Could you check a few things on this model? Use its own coordinates, in mm. Face numbers are marked on the shaded views. A direction names the side the tool comes from. Give positions to 0.01 mm unless a question says otherwise; leave off trailing zeros. Write each loop counter-clockwise with the first axis right and the second up, starting at its lowest first coordinate (ties: lowest second). Pieces come first, ordered by that corner, then holes. Notation, with made-up numbers: (11.25, 68) - (53.25, 68) arc R19 cw to (53.25, 96) - close; hole circle Ø3 at (80.25, 44.25). An arc over 180 degrees is marked (long way). Write item = value, one per line.
from build123d import *

# Parameters (mm, degrees)
SKETCH1_R           = 1.6
BOSS_EXTRUDE1_DEPTH = 5
BOSS_EXTRUDE2_DEPTH = 79.5
SKETCH3_R           = 11.1
CUT_EXTRUDE1_DEPTH  = 112.08808442
BOSS_EXTRUDE3_START = 3
SKETCH4_R           = 15
SKETCH4_R_2         = 11.1
BOSS_EXTRUDE3_DEPTH = 3
CHAMFER1_SIZE       = 3
BOSS_EXTRUDE4_START = -1
SKETCH5_R           = 11.1
SKETCH5_R_2         = 9.1
BOSS_EXTRUDE4_DEPTH = 1
CHAMFER2_SIZE       = 10
CHAMFER2_SIZE_2     = 0.5
SKETCH6_R           = 1.6
CUT_EXTRUDE2_DEPTH  = 112.08808442
SKETCH7_R           = 11.1
SKETCH7_R_2         = 1.6
CUT_EXTRUDE3_DEPTH  = 112.995814654
BOSS_EXTRUDE5_START = -1
SKETCH8_R           = 11.1
SKETCH8_R_2         = 9.1
BOSS_EXTRUDE5_DEPTH = 1
CHAMFER3_SIZE       = 10
CHAMFER3_SIZE_2     = 0.5
BOSS_EXTRUDE6_START = 5.5
SKETCH9_R           = 1.6
SKETCH9_R_2         = 11.1
BOSS_EXTRUDE6_DEPTH = 5.5
SKETCH10_R          = 12.5
CUT_EXTRUDE4_DEPTH  = 2.5
CHAMFER6_SIZE       = 1
CHAMFER5_SIZE       = 5.5
FILLET4_R           = 5
FILLET5_R           = 5
FILLET6_R           = 5
FILLET7_R           = 5
FILLET1_R           = 10


# Some blends are built 0.0001 mm under size
with BuildPart() as part:
    # Sketch1 → Boss-Extrude1 (new body)
    with BuildSketch(Plane.XY):
        with BuildLine():
            Line((-32.25, -32.25), (-16.996827309, -32.25))
            ThreePointArc((-16.996827309, -32.25), (-13.644608083, -30.959801378), (-12.022400308, -27.755050505))
            ThreePointArc((-12.022400308, -27.755050505), (0.783748237, -0.783748237), (27.755050505, 12.022400308))
            ThreePointArc((27.755050505, 12.022400308), (30.959801378, 13.644608083), (32.25, 16.996827309))
            Line((32.25, 16.996827309), (32.25, 32.25))
            Line((32.25, 32.25), (-32.25, 32.25))
            Line((-32.25, 32.25), (-32.25, -32.25))
        make_face()
        with Locations((-19.75, 19.75)):
            Circle(SKETCH1_R, mode=Mode.SUBTRACT)
        with Locations((-5.65, 19.75)):
            Circle(SKETCH1_R, mode=Mode.SUBTRACT)
        with Locations((25.65, 19.75)):
            Circle(SKETCH1_R, mode=Mode.SUBTRACT)
        with Locations((-19.75, 5.65)):
            Circle(SKETCH1_R, mode=Mode.SUBTRACT)
        with Locations((-19.75, -25.65)):
            Circle(SKETCH1_R, mode=Mode.SUBTRACT)
    extrude(amount=BOSS_EXTRUDE1_DEPTH)

    # Sketch2 → Boss-Extrude2 (add)
    with BuildSketch(Plane.XY.offset(5)):
        Polygon((-32.25, 32.25), (32.25, 32.25), (32.25, 27.25), (-27.25, 27.25), (-27.25, -32.25), (-32.25, -32.25), (-32.25, 27.25), align=None)
    extrude(amount=BOSS_EXTRUDE2_DEPTH)

    # Sketch3 → Cut-Extrude1 (cut, through all)
    with BuildSketch(Plane(origin=(0, 32.25, 0), x_dir=(1, 0, 0), z_dir=(0, 1, 0))):
        with Locations(Location((11.85, -64.1, 0), (0, 0, 270))):
            Circle(SKETCH3_R)
        with BuildLine():
            Line((11.85, -84.5), (11.85, -91.476631288))
            Line((11.85, -91.476631288), (44.100409765, -91.476631288))
            Line((44.100409765, -91.476631288), (44.100409765, -64.1))
            Line((44.100409765, -64.1), (32.25, -64.1))
            ThreePointArc((32.25, -64.1), (26.274978336, -78.524978336), (11.85, -84.5))
        make_face()
    extrude(amount=-CUT_EXTRUDE1_DEPTH, mode=Mode.SUBTRACT)

    # Sketch4 → Boss-Extrude3 (add)
    with BuildSketch(Plane(origin=(0, 32.25, 0), x_dir=(1, 0, 0), z_dir=(0, 1, 0)).offset(BOSS_EXTRUDE3_START)):
        with Locations(Location((11.85, -64.1, 0), (0, 0, 90))):
            Circle(SKETCH4_R)
        with Locations(Location((11.85, -64.1, 0), (0, 0, 270))):
            Circle(SKETCH4_R_2, mode=Mode.SUBTRACT)
    extrude(amount=-BOSS_EXTRUDE3_DEPTH)

    # Chamfer1
    chamfer1_edges = [part.edges().sort_by_distance(p)[0] for p in [
        (11.85, 35.25, 79.1),
    ]]
    chamfer(chamfer1_edges, length=CHAMFER1_SIZE - 0.0001)  # a hair under: the kernel refuses the full size

    # Sketch5 → Boss-Extrude4 (add)
    with BuildSketch(Plane.XZ.offset(-27.25).offset(BOSS_EXTRUDE4_START)):
        with Locations(Location((11.85, 64.1, 0), (0, 0, 90))):
            Circle(SKETCH5_R)
        with Locations(Location((11.85, 64.1, 0), (0, 0, 270))):
            Circle(SKETCH5_R_2, mode=Mode.SUBTRACT)
    extrude(amount=BOSS_EXTRUDE4_DEPTH)

    # Chamfer2
    # the kernel refuses this chamfer: 10, 0.5 mm, written as the material it takes off along each edge
    with BuildSketch(Plane(origin=(11.85, 28.25, 64.1), x_dir=(0, 0, -1), z_dir=(-1, 0, 0))) as chamfer2_piece_1_section:
        Polygon((9.1 + CHAMFER2_SIZE, 0), (9.1, CHAMFER2_SIZE_2), (9.1, 0), align=None)
    chamfer2_piece_1 = revolve(axis=Axis((11.85, 28.25, 64.1), (0, -1, 0)), mode=Mode.PRIVATE)
    chamfer2_piece_1 = chamfer2_piece_1 & Plane(origin=(11.85, 27.834786479, 64.1), x_dir=(0, 0, 1), z_dir=(0, 1, 0)) * Cylinder(11.1, 77, mode=Mode.PRIVATE)
    add(chamfer2_piece_1, mode=Mode.SUBTRACT)

    # Sketch6 → Cut-Extrude2 (cut, through all)
    with BuildSketch(Plane(origin=(0, 32.25, 0), x_dir=(1, 0, 0), z_dir=(0, 1, 0))):
        with Locations(Location((-19.75, -26.6, 0), (0, 0, 270))):
            Circle(SKETCH6_R)
        with Locations(Location((-19.75, -77.9, 0), (0, 0, 270))):
            Circle(SKETCH6_R)
        with Locations(Location((-5.65, -12.5, 0), (0, 0, 270))):
            Circle(SKETCH6_R)
        with Locations(Location((25.65, -12.5, 0), (0, 0, 270))):
            Circle(SKETCH6_R)
    extrude(amount=-CUT_EXTRUDE2_DEPTH, mode=Mode.SUBTRACT)

    # Sketch7 → Cut-Extrude3 (cut, through all)
    with BuildSketch(Plane.ZY.offset(32.25)):
        with Locations((44.1, -11.85)):
            Circle(SKETCH7_R)
        with Locations((28.6, -27.35)):
            Circle(SKETCH7_R_2)
        with Locations((57.9, 19.75)):
            Circle(SKETCH7_R_2)
        with Locations((26.6, 19.75)):
            Circle(SKETCH7_R_2)
        with Locations((12.5, 5.65)):
            Circle(SKETCH7_R_2)
        with Locations((12.5, -25.65)):
            Circle(SKETCH7_R_2)
        with Locations((28.6, 3.65)):
            Circle(SKETCH7_R_2)
        with Locations((59.6, 3.65)):
            Circle(SKETCH7_R_2)
        with Locations((59.6, -27.35)):
            Circle(SKETCH7_R_2)
        with BuildLine():
            Line((64.5, -32.25), (64.5, 19.75))
            ThreePointArc((64.5, 19.75), (66.696699141, 25.053300859), (72, 27.25))
            Line((72, 27.25), (84.5, 27.25))
            Line((84.5, 27.25), (84.5, -32.25))
            Line((84.5, -32.25), (64.5, -32.25))
        make_face()
    extrude(amount=-CUT_EXTRUDE3_DEPTH, mode=Mode.SUBTRACT)

    # Sketch8 → Boss-Extrude5 (add)
    with BuildSketch(Plane(origin=(-27.25, 0, 0), x_dir=(0, 0, -1), z_dir=(1, 0, 0)).offset(BOSS_EXTRUDE5_START)):
        with Locations(Location((-44.1, -11.85, 0), (0, 0, 180))):
            Circle(SKETCH8_R)
        with Locations(Location((-44.1, -11.85, 0), (0, 0, 90))):
            Circle(SKETCH8_R_2, mode=Mode.SUBTRACT)
    extrude(amount=BOSS_EXTRUDE5_DEPTH)

    # Chamfer3
    # the kernel refuses this chamfer: 10, 0.5 mm, written as the material it takes off along each edge
    with BuildSketch(Plane(origin=(-28.25, -11.85, 44.1), x_dir=(0, 1, 0), z_dir=(0, 0, -1))) as chamfer3_piece_1_section:
        Polygon((9.1 + CHAMFER3_SIZE, 0), (9.1, CHAMFER3_SIZE_2), (9.1, 0), align=None)
    chamfer3_piece_1 = revolve(axis=Axis((-28.25, -11.85, 44.1), (1, 0, 0)), mode=Mode.PRIVATE)
    chamfer3_piece_1 = chamfer3_piece_1 & Plane(origin=(-27.834786479, -11.85, 44.1), x_dir=(0, 0, 1), z_dir=(-1, 0, 0)) * Cylinder(11.1, 77, mode=Mode.PRIVATE)
    add(chamfer3_piece_1, mode=Mode.SUBTRACT)

    # Sketch9 → Boss-Extrude6 (add)
    with BuildSketch(Plane.ZY.offset(32.25).offset(BOSS_EXTRUDE6_START)):
        Polygon((64.5, -32.25), (23.7, -32.25), (18.2, -32.25), (18.2, 8.55), (23.7, 8.55), (64.5, 8.55), align=None)
        with Locations((28.6, -27.35)):
            Circle(SKETCH9_R, mode=Mode.SUBTRACT)
        with Locations((28.6, 3.65)):
            Circle(SKETCH9_R, mode=Mode.SUBTRACT)
        with Locations((44.1, -11.85)):
            Circle(SKETCH9_R_2, mode=Mode.SUBTRACT)
        with Locations((59.6, 3.65)):
            Circle(SKETCH9_R, mode=Mode.SUBTRACT)
        with Locations((59.6, -27.35)):
            Circle(SKETCH9_R, mode=Mode.SUBTRACT)
    extrude(amount=-BOSS_EXTRUDE6_DEPTH)

    # Sketch10 → Cut-Extrude4 (cut)
    with BuildSketch(Plane.ZY.offset(37.75)):
        with Locations((44.1, -11.85)):
            Circle(SKETCH10_R)
    extrude(amount=-CUT_EXTRUDE4_DEPTH, mode=Mode.SUBTRACT)

    # Chamfer6
    chamfer6_edges = [part.edges().sort_by_distance(p)[0] for p in [
        (-37.75, -11.85, 31.6),
    ]]
    chamfer(chamfer6_edges, length=CHAMFER6_SIZE)

    # Chamfer5
    chamfer5_edges = [part.edges().sort_by_distance(p)[0] for p in [
        (-37.75, -11.85, 18.2),
    ]]
    chamfer(chamfer5_edges, length=CHAMFER5_SIZE - 0.0001)  # a hair under: the kernel refuses the full size

    # Fillet4
    fillet4_edges = [part.edges().sort_by_distance(p)[0] for p in [
        (-32.5, -32.25, 64.5),
    ]]
    fillet(fillet4_edges, radius=FILLET4_R)

    # Fillet5
    fillet5_edges = [part.edges().sort_by_distance(p)[0] for p in [
        (-35, 8.55, 64.5),
    ]]
    fillet(fillet5_edges, radius=FILLET5_R)

    # Fillet6
    fillet6_edges = [part.edges().sort_by_distance(p)[0] for p in [
        (-35.00005, 8.55, 20.94995),
    ]]
    fillet(fillet6_edges, radius=FILLET6_R)

    # Fillet7
    # the kernel refuses this fillet: 5 mm, written as the material it takes off along each edge
    with BuildSketch(Plane(origin=(-46.588834765, -32.25, 32.538734765), x_dir=(0, 1, 0), z_dir=(0.7071067811865478, 0, -0.7071067811865474))) as fillet7_piece_1_section:
        with BuildLine():
            CenterArc((FILLET7_R, FILLET7_R), FILLET7_R, 180, 90)
            Line((0, FILLET7_R), (0, 0))
            Line((0, 0), (FILLET7_R, 0))
        make_face()
    fillet7_piece_1 = extrude(amount=32.778033172, mode=Mode.PRIVATE)
    fillet7_piece_1 = split(fillet7_piece_1, bisect_by=Plane(origin=(-32.25, -31.133160306, 22.529349846), z_dir=(-1, 0, 0)), keep=Keep.TOP, mode=Mode.PRIVATE)
    add(fillet7_piece_1, mode=Mode.SUBTRACT)

    # Fillet1
    fillet1_edges = [part.edges().sort_by_distance(p)[0] for p in [
        (-32.25, 29.75, 84.5),
    ]]
    fillet(fillet1_edges, radius=FILLET1_R)


solid = part.part
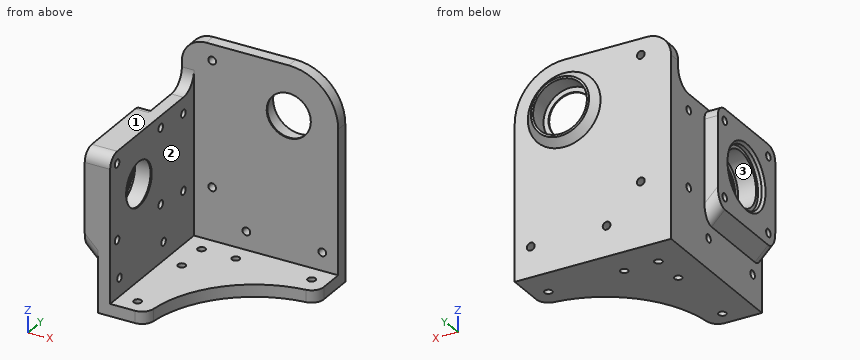
1. For pin 1 (5 mm diameter, centred on x = -33.5, y = -13, fed in from +Z); pin 2 (3 mm diameter, centred on x = -19.75, z = 26.6, fed in from +Y); pin 3 (3.5 mm diameter, centred on y = 5.65, z = 12.5, fed in from -X); pin 4 (23.5 mm diameter, centred on y = -11.85, z = 44.1, fed in from -X), each with a flat end and sliding along its axis, tell me the tip position at first contact or that it passes through.
Filled sheet:
pin_1 = 64.5
pin_2 = through
pin_3 = -32.25
pin_4 = -35.25
2. I need wall thicknesses on line 1 (Z direction, x = -29, y = 3); line 2 (Y direction, x = -19, z = 2); line 3 (X direction, y = 27.45, z = 64.1). Which ranges of each line are inside material? Lowest first, please.
Filled sheet:
line_1 = 0 to 27.14, 30.06 to 58.14, 61.06 to 64.5
line_2 = -32.25 to -27.06, -24.24 to 4.24, 7.06 to 18.34, 21.16 to 32.25
line_3 = -32.25 to 2.75, 20.95 to 32.25
3. Which directions (+Z, -Z, +X, -X, +Y, -Y) give clear straight access to the entire face, cutting with the end or side of a thin tool? Please do the marked faces 1, 2 and 3.
Filled sheet:
face_1 = +Z, +X, -X, -Y
face_2 = +Z, +X, -Y
face_3 = -X
4. If we section it at A-A, the plane x = -5.65: Please give me the cut outline in (y, z), and give its area (3 significant figures).
Filled sheet:
outline = (-8.93, 0) - (18.15, 0) - (18.15, 5) - (-8.93, 5) - close; (21.35, 0) - (32.25, 0) - (32.25, 10.9) - (27.25, 10.9) - (27.25, 5) - (21.35, 5) - close; (27.25, 14.1) - (32.25, 14.1) - (32.25, 84.5) - (27.25, 84.5) - close
area = 571 mm2
5. If we section it at C-C, the plane y = 24.5: Please give me the cut outline in (x, z), and give its area (3 significant figures).
Filled sheet:
outline = (-32.25, 0) - (32.25, 0) - (32.25, 5) - (-27.25, 5) - (-27.25, 66.2) - (-32.25, 66.2) - close
area = 628 mm2
6. If we section it at B-B, the plane y = 14: Please give me the cut outline in (x, z).
Filled sheet:
outline = (-32.25, 0) - (31.25, 0) - (31.25, 5) - (-27.25, 5) - (-27.25, 64.5) - (-32.25, 64.5) - close
